The model under review builds one solid part; all positions refer to its coordinate system, in mm. Face numbers are marked on the shaded views. A direction names the side the tool comes from. Round coordinates to 2 decimals unless told otherwise and drop trailing zeros. Loops run counter-clockwise (first coordinate to the right, second up) from the corner with the lowest first, then second, coordinate; pieces in that order, holes last. Notation, with made-up numbers: (-31.75, 28.5) -> (20.25, 28.5) arc R11 ccw to (20.25, 38.5) -> close; hole circle Ø2 at (36.25, -26.75). An arc over 180 degrees is marked (long way). Use a Markdown table: item, result. Add a question column.
1) Consider section D-D on z = 28.5. Give the boundary of the cut face in (x, y).
2) Consider section A-A on x = 0. Give the boundary of the cut face in (y, z), plus the area to 3 significant figures.
3) Consider section C-C on z = 103. Give the boundary of the cut face in (x, y), plus the area to 3 significant figures.
4) Wall thickness on probe 1 along Z at (x, y) = (8, 2.5); probe 2 along X at (y, z) = (1.5, 38); probe 3 along Z at (x, y) = (-7.5, -29.5): over which ranges is each line inside the solid? List them lowest first.
5) Insertion check: pin 1 (1 mm diameter, centred on x = -21, z = 27.5, fed in from +Y); pin 2 (1.5 mm diameter, centred on x = -4.5, y = 21, fed in from +Z); pin 3 (6 mm diameter, centred on y = 2, z = 72, fed in from -X). Each pin has a flat end and moves straight along its axis. Give the tip position at first contact, or say it passes through.
6) For the marked faces 1 and 2, list the 3-axis set-ups (+Z, -Z, +X, -X, +Y, -Y) from which the entire face can be reached by the end or side of a thin tool; tool diameter is ignored.
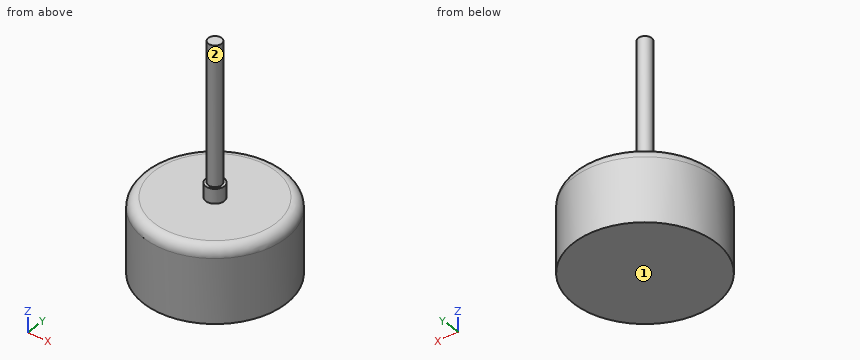
from build123d import *

# Parameters (mm, degrees)
F1_R     = 3.25
F3_DEPTH = 110
F0_R     = 34.5
F4_DEPTH = 36
F2_R     = 4.5
F5_DEPTH = 43
F6_R     = 5


with BuildPart() as f3:
    # F1 (on Top) → F3 (new body)
    with BuildSketch(Plane.XY):
        Circle(F1_R)
    extrude(amount=F3_DEPTH)

    # F0 (on Top) → F4 (join)
    with BuildSketch(Plane.XY):
        Circle(F0_R)
    extrude(amount=F4_DEPTH)

    # F2 (on Top) → F5 (join)
    with BuildSketch(Plane.XY):
        Circle(F2_R)
    extrude(amount=F5_DEPTH)

    # F6
    f6_edges = [f3.edges().sort_by_distance(p)[0] for p in [
        (-34.5, 0, 36),
    ]]
    fillet(f6_edges, radius=F6_R)


solid = f3.part
Result set:
| question | item | result |
|---|---|---|
| 1 | outline | circle Ø69 at (0, 0) |
| 2 | outline | (-34.5, 0) -> (34.5, 0) -> (34.5, 31) arc R5 ccw to (29.5, 36) -> (4.5, 36) -> (4.5, 43) -> (3.25, 43) -> (3.25, 110) -> (-3.25, 110) -> (-3.25, 43) -> (-4.5, 43) -> (-4.5, 36) -> (-29.5, 36) arc R5 ccw to (-34.5, 31) -> close |
| 2 | area | 2,970 mm2 |
| 3 | outline | circle Ø6.5 at (0, 0) |
| 3 | area | 33.2 mm2 |
| 4 | probe 1 | 0 to 36 |
| 4 | probe 2 | -4.24 to 4.24 |
| 4 | probe 3 | 0 to 35.91 |
| 5 | pin 1 | y = 27.75 |
| 5 | pin 2 | z = 36 |
| 5 | pin 3 | x = -3.25 |
| 6 | face 1 | -Z, +X, -X, +Y, -Y |
| 6 | face 2 | +Z |
